The model under review builds one solid part; all positions refer to its coordinate system, in mm. Face numbers are marked on the shaded views. A direction names the side the tool comes from. Give positions to 0.01 mm unless a question says otherwise; leave off trailing zeros. Loops run counter-clockwise (first coordinate to the right, second up) from the corner with the lowest first, then second, coordinate; pieces in that order, holes last. Notation, with made-up numbers: (43, 89) - (100, 89) arc R27 cw to (100, 116) - close; hole circle Ø11 at (69.5, -22.75). An arc over 180 degrees is marked (long way). Return JSON: item names as keys, results as strings. Group by question number.
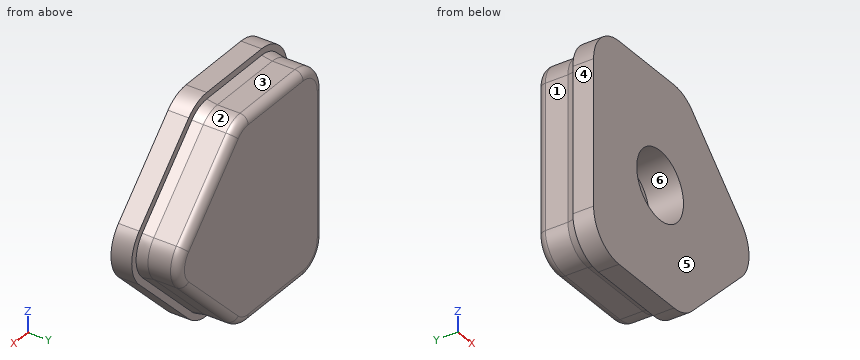
from build123d import *

# Parameters (mm, degrees)
EXTRUDE_3_DEPTH     = 1
EXTRUDE_4_DEPTH     = 2
CHAMFER_1_SIZE      = 0.09
CHAMFER_1_SIZE2     = 0.510415364
FILLET_3_R          = 0.4
SKETCH_8_R          = 1.65
CUT_EXTRUDE_1_DEPTH = 1.65


with BuildPart() as part:
    # 草图5 → 凸台-拉伸3 (new body)
    with BuildSketch(Plane(origin=(0, 0, 0), x_dir=(1, 0, 0), z_dir=(0, 1, 0))):
        with BuildLine():
            Line((-4.5, -5.3), (-0.621320344, -5.3))
            ThreePointArc((-0.621320344, -5.3), (0.067509835, -5.162983159), (0.651471863, -4.772792206))
            Line((0.651471863, -4.772792206), (4.151471863, -1.272792206))
            ThreePointArc((4.151471863, -1.272792206), (4.678679656, 0), (4.151471863, 1.272792206))
            Line((4.151471863, 1.272792206), (0.651471863, 4.772792206))
            ThreePointArc((0.651471863, 4.772792206), (0.067509835, 5.162983159), (-0.621320344, 5.3))
            Line((-0.621320344, 5.3), (-4.5, 5.3))
            ThreePointArc((-4.5, 5.3), (-5.772792206, 4.772792206), (-6.3, 3.5))
            Line((-6.3, 3.5), (-6.3, -3.5))
            ThreePointArc((-6.3, -3.5), (-5.772792206, -4.772792206), (-4.5, -5.3))
        make_face()
    extrude(amount=EXTRUDE_3_DEPTH)

    # 草图6 → 凸台-拉伸4 (add)
    with BuildSketch(Plane(origin=(0, 1, 0), x_dir=(1, 0, 0), z_dir=(0, 1, 0))):
        with BuildLine():
            Line((-4.5, -4.9), (-0.621320344, -4.9))
            ThreePointArc((-0.621320344, -4.9), (-0.085563538, -4.793431346), (0.36862915, -4.489949494))
            Line((0.36862915, -4.489949494), (3.86862915, -0.989949494))
            ThreePointArc((3.86862915, -0.989949494), (4.278679656, 0), (3.86862915, 0.989949494))
            Line((3.86862915, 0.989949494), (0.36862915, 4.489949494))
            ThreePointArc((0.36862915, 4.489949494), (-0.085563538, 4.793431346), (-0.621320344, 4.9))
            Line((-0.621320344, 4.9), (-4.5, 4.9))
            ThreePointArc((-4.5, 4.9), (-5.489949494, 4.489949494), (-5.9, 3.5))
            Line((-5.9, 3.5), (-5.9, -3.5))
            ThreePointArc((-5.9, -3.5), (-5.489949494, -4.489949494), (-4.5, -4.9))
        make_face()
    extrude(amount=EXTRUDE_4_DEPTH)

    # 倒角1
    chamfer_1_edges = [part.edges().sort_by_distance(p)[0] for p in [
        (-5.489949494, 1, 4.489949494),
        (-2.560660172, 1, 4.9),
        (-0.085563538, 1, 4.793431346),
        (2.11862915, 1, 2.739949494),
        (4.278679656, 1, 0),
        (2.11862915, 1, -2.739949494),
        (-0.085563538, 1, -4.793431346),
        (-2.560660172, 1, -4.9),
        (-5.489949494, 1, -4.489949494),
        (-5.9, 1, 0),
    ]]
    chamfer_1_side = [part.faces().sort_by_distance(p)[0] for p in [
        (-2.560660172, 1, 5.1473922),
    ]]
    chamfer(chamfer_1_edges, length=CHAMFER_1_SIZE, length2=CHAMFER_1_SIZE2, reference=chamfer_1_side[0])

    # 圆角3
    fillet_3_edges = [part.edges().sort_by_distance(p)[0] for p in [
        (-5.489949494, 3, 4.489949494),
        (-2.560660172, 3, 4.9),
        (-0.085563538, 3, 4.793431346),
        (2.11862915, 3, 2.739949494),
        (4.278679656, 3, 0),
        (2.11862915, 3, -2.739949494),
        (-0.085563538, 3, -4.793431346),
        (-2.560660172, 3, -4.9),
        (-5.489949494, 3, -4.489949494),
        (-5.9, 3, 0),
    ]]
    fillet(fillet_3_edges, radius=FILLET_3_R)

    # 草图8 → 切除-拉伸1 (cut)
    with BuildSketch(Plane.XZ):
        with Locations((-1.6, 0)):
            Circle(SKETCH_8_R)
    extrude(amount=-CUT_EXTRUDE_1_DEPTH, mode=Mode.SUBTRACT)


solid = part.part
Item 1: Take a section at B-B (x = -1.6). State the section outline as (y, z) points, then the cut area to 3 significant figures.
Item 2: Take a section at D-D (z = 0). State the section outline as (x, y) points, then the cut area to 3 significant figures.
Item 3: Take a section at A-A (y = 0.8). State the section outline as (x, z) points, then the cut area to 3 significant figures.
Item 4: For P1, Ø1.5, axis at y = 2.5, z = 3, coming from the -X side; P2, Ø0.9, axis at x = -2.5, y = 2, coming from the -Z side; P3, Ø1.2, axis at x = -3.5, y = 2, coming from the +Z side, all flat-tipped, find the tip position at first contact; note any pin that passes through.
Item 5: Mouldability with a two-part tool opening along X and no side actions: class the marked faces 4, 5 and 6 as +X half, -X half, draft (parallel to the pull), parting line (faces both ways), or undercut.
Item 6: Take a section at C-C (y = 2.45). State the section outline as (x, z) points.
Item 7: For L1, parallel to Z at x = -1.6, y = 0.55; L2, parallel to Z at x = -2.5, y = 2.05; L3, parallel to Y at x = -2, z = -1.5, list the stretches that pass through material, from the lowest coordinate up. Write a range as from..to.
Item 8: Tool access review of the marked faces 1, 2 and 3: name each direction out of +Z, -Z, +X, -X, +Y, -Y from which nothing blocks a thin tool from reaching the whole face with its end or side.
Check sheet entries:
{
 "1": {"outline": "(0, -5.3) - (1, -5.3) - (1, -4.99) - (1.51, -4.9) - (2.6, -4.9) arc R0.4 ccw to (3, -4.5) - (3, 4.5) arc R0.4 ccw to (2.6, 4.9) - (1.51, 4.9) - (1, 4.99) - (1, 5.3) - (0, 5.3) - (0, 1.65) - (1.65, 1.65) - (1.65, -1.65) - (0, -1.65) - close", "area": "24.7 mm^2"},
 "2": {"outline": "(-6.3, 0) - (-3.25, 0) - (-3.25, 1.65) - (0.05, 1.65) - (0.05, 0) - (4.68, 0) - (4.68, 1) - (4.37, 1) - (4.28, 1.51) - (4.28, 2.6) arc R0.4 ccw to (3.88, 3) - (-5.5, 3) arc R0.4 ccw to (-5.9, 2.6) - (-5.9, 1.51) - (-5.99, 1) - (-6.3, 1) - close", "area": "25.9 mm^2"},
 "3": {"outline": "(-6.3, -3.5) arc R1.8 ccw to (-4.5, -5.3) - (-0.62, -5.3) arc R1.8 ccw to (0.65, -4.77) - (4.15, -1.27) arc R1.8 ccw to (4.15, 1.27) - (0.65, 4.77) arc R1.8 ccw to (-0.62, 5.3) - (-4.5, 5.3) arc R1.8 ccw to (-6.3, 3.5) - close; hole circle Ø3.3 at (-1.6, 0)", "area": "85.4 mm^2"},
 "4": {"P1": "stops at x = -5.9", "P2": "stops at z = -4.9", "P3": "stops at z = 4.92"},
 "5": {"face 4": "-X half", "face 5": "draft", "face 6": "undercut"},
 "6": {"outline": "(-5.9, -3.5) arc R1.4 ccw to (-4.5, -4.9) - (-0.62, -4.9) arc R1.4 ccw to (0.37, -4.49) - (3.87, -0.99) arc R1.4 ccw to (3.87, 0.99) - (0.37, 4.49) arc R1.4 ccw to (-0.62, 4.9) - (-4.5, 4.9) arc R1.4 ccw to (-5.9, 3.5) - close"},
 "7": {"L1": "z = -5.3..-1.65, 1.65..5.3", "L2": "z = -4.9..4.9", "L3": "y = 1.65..3"},
 "8": {"face 1": "+Z, -Z, -X, +Y", "face 2": "+Z, +X, +Y", "face 3": "+Z, +X, -X, +Y"}
}
